Geometry: see drawing. Coordinates: mm, zero at the bounding-box minimum. A direction names the side the tool comes from. Coordinates: 2 decimals unless noted, no trailing zeros. Write each loop counter-clockwise with the first axis right and the second up, starting at its lowest first coordinate (ties: lowest second). Pieces come first, ordered by that corner, then holes. Notation, with made-up numbers: (-24, 79) -> (35, 79) arc R20 cw to (35, 88) -> close; hole circle Ø6 at (7.25, 22). An arc over 180 degrees is marked (long way). Use one line per item in the form item = value. Start each with the question number.
(1) Cut plane C-C on y = 14. Return the cut outline in (x, z), plus the area to 3 significant figures.
(2) Cut plane D-D on x = 46. Return the cut outline in (y, z).
(3) First-contact query: pin 1 (2 mm diameter, centred on y = 46, z = 23.5, fed in from -X); pin 2 (4 mm diameter, centred on y = 44, z = 38, fed in from +X); pin 3 (18 mm diameter, centred on x = 34, y = 43.5, fed in from +Z); pin 4 (8 mm diameter, centred on y = 24.5, z = 42, fed in from -X). Flat tips, straight axial feed; report the tip coordinate or a pass-through.
(4) Cut plane B-B on x = 30. Return the cut outline in (y, z).
(5) Cut plane A-A on z = 27.5. Return the cut outline in (x, y), plus the area to 3 significant figures.
(6) Ray query, line 1 along X through (y, z) = (25, 20); line 2 along Z through (x, y) = (30.5, 13); line 3 along Z through (x, y) = (35, 45). Return the intervals inside material, ascending.
(7) Set-up query: the marked faces 5, 6 and 7. Return all of +Z, -Z, +X, -X, +Y, -Y with unobstructed straight access to the full face (end or side cutting, diameter ignored); none if empty.
(8) Pull-direction query (Z, two-part tool) for the marked faces 1, 2, 3 and 4; classes: released by +Z, released by -Z, zero draft, split by the parting line, or undercut.
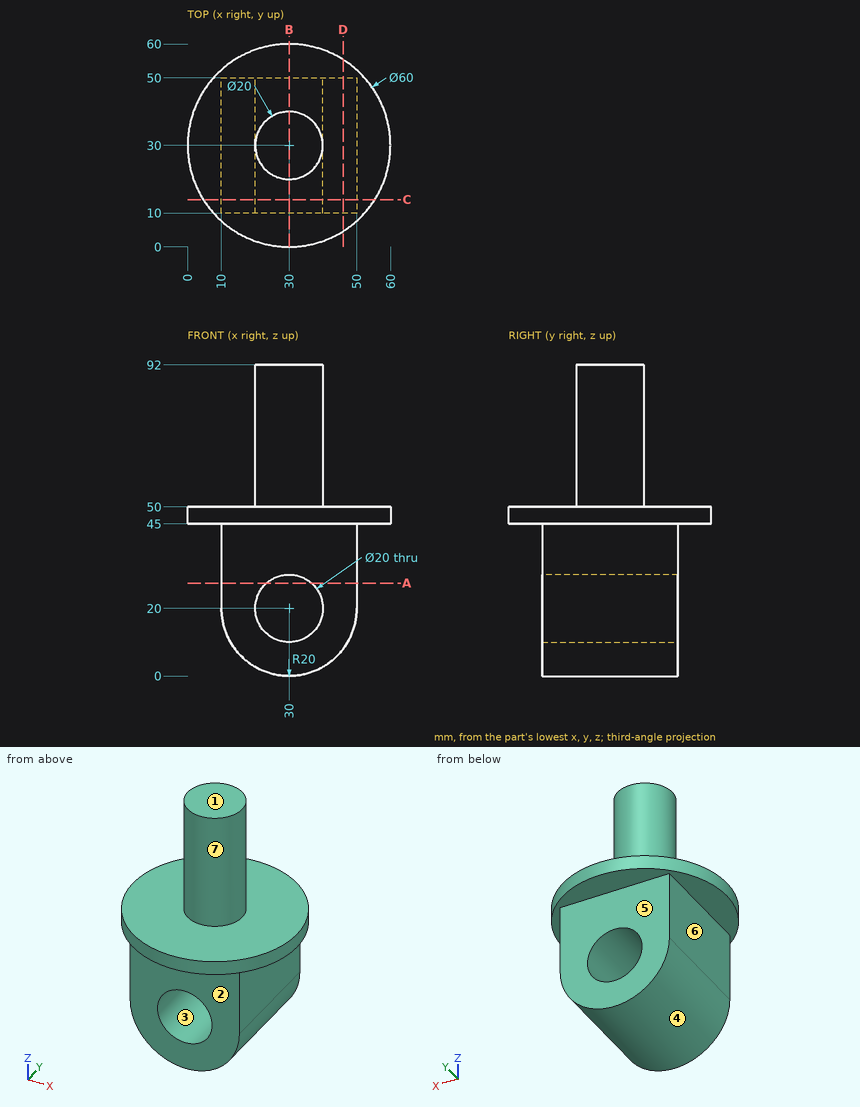
Values:
q1.outline = (4.62, 45) -> (10, 45) -> (10, 20) arc R20 ccw to (50, 20) -> (50, 45) -> (55.38, 45) -> (55.38, 50) -> (4.62, 50) -> close; hole circle Ø20 at (30, 20)
q1.area = 1,570 mm2
q2.outline = (4.62, 45) -> (10, 45) -> (10, 8) -> (50, 8) -> (50, 45) -> (55.38, 45) -> (55.38, 50) -> (4.62, 50) -> close
q3.pin_1 = 10
q3.pin_2 = 50
q3.pin_3 = 92
q3.pin_4 = 0.14
q4.outline = (0, 45) -> (10, 45) -> (10, 30) -> (50, 30) -> (50, 45) -> (60, 45) -> (60, 50) -> (40, 50) -> (40, 92) -> (20, 92) -> (20, 50) -> (0, 50) -> close; (10, 0) -> (50, 0) -> (50, 10) -> (10, 10) -> close
q5.outline = (10, 10) -> (23.39, 10) -> (23.39, 50) -> (10, 50) -> close; (36.61, 10) -> (50, 10) -> (50, 50) -> (36.61, 50) -> close
q5.area = 1,070 mm2
q6.line_1 = 10 to 20, 40 to 50
q6.line_2 = 0.01 to 10.01, 29.99 to 50
q6.line_3 = 0.64 to 11.34, 28.66 to 50
q7.face_5 = -Z, +X, -X, +Y
q7.face_6 = -Z, -X, +Y, -Y
q7.face_7 = +Z
q8.face_1 = released by +Z
q8.face_2 = zero draft
q8.face_3 = undercut
q8.face_4 = released by -Z
